Verification items for the finished model (mm, model axes). Round coordinates to 2 decimals unless told otherwise and drop trailing zeros. Order: outer loops, then holes, each group sorted by start corner. A loop starts at its lowest first (then second) coordinate and runs counter-clockwise, first axis right, second up. Notation, with made-up numbers: M -22,71 L 20,71 A30 ccw 20,108 Z; hole C 68.25,80 d3. An arc over 180 degrees is marked long. Use CSV: the item, a comma, the result in double quotes. Start each with the question number.
Q1. Sectioned sample at D-D (z = -51). Enter the section's corners in (x, y).
Q2. Mould release check, pull along X, two halves, no side actions. Record for faces 1 (the face through (-10.867, 82.767, -77.244)), 2 (the face through (0.501, 76.326, 14.743)), 3 (the face through (-25.94, 68.03, 34.57)): +X half, -X half, draft (parallel to the pull), parting line (faces both ways), or undercut.
Q3. Sectioned sample at C-C (y = 8.5). Enter the section's corners in (x, z).
Q4. Sectioned sample at A-A (x = 0). Enter the section's corners in (y, z), and give its area (3 significant figures).
Q5. Gauge pin test, flat ends, axial feed: pin 1 Ø1 at (y, z) = (43, -75) entering from +X; pin 2 Ø10 at (x, z) = (42.5, -95.5) entering from +Y; pin 3 Ø10 at (y, z) = (-30, -48) entering from -X. Record the tip position at first contact, or that the pin passes through.
Q6. Sectioned sample at B-B (y = -23). Enter the section's corners in (x, z).
Q7. Scan lines: line 1 (Y direction, x = -9.5, z = -155); line 2 (Y direction, x = 0, z = -107.5); line 3 (Y direction, x = -24, z = -144). Record each from-to range of solid material in increasing order.
```python
from build123d import *

# Parameters (mm, degrees)
SKETCH1_R                = 83.4771
SKETCH1_R_2              = 72.5043
BOSS_EXTRUDE1_DEPTH      = 203.2
BOSS_EXTRUDE1_DEPTH_BACK = 177.8
SKETCH8_W                = 2032
SKETCH8_H                = 2032
CUT_EXTRUDE10_DEPTH      = 304.8
SKETCH17_W               = 203.2
SKETCH17_H               = 508
CUT_EXTRUDE14_DEPTH      = 152.4
SKETCH18_R               = 25.4
CUT_EXTRUDE15_DEPTH      = 238.393289234


with BuildPart() as part:
    # Sketch1 → Boss-Extrude1 (new body, two sides)
    with BuildSketch(Plane.XY) as boss_extrude1_sk:
        Circle(SKETCH1_R)
        Circle(SKETCH1_R_2, mode=Mode.SUBTRACT)
    extrude(amount=BOSS_EXTRUDE1_DEPTH)
    extrude(boss_extrude1_sk.sketch, amount=-BOSS_EXTRUDE1_DEPTH_BACK)

    # Sketch8 → Cut-Extrude10 (cut)
    with BuildSketch(Plane(origin=(0, 0, 0), x_dir=(-1, 0, 0), z_dir=(0, 0.866025404, -0.5))):
        Rectangle(SKETCH8_W, SKETCH8_H)
    extrude(amount=-CUT_EXTRUDE10_DEPTH, mode=Mode.SUBTRACT)

    # Sketch17 → Cut-Extrude14 (cut)
    with BuildSketch(Plane(origin=(0, 65.991135768, 38.1), x_dir=(-1, 0, 0), z_dir=(0, 0.866025404, 0.5))):
        Rectangle(SKETCH17_W, SKETCH17_H)
    extrude(amount=CUT_EXTRUDE14_DEPTH, mode=Mode.SUBTRACT)

    # Sketch18 → Cut-Extrude15 (cut, through all)
    with BuildSketch(Plane(origin=(0, 65.991135768, 38.1), x_dir=(1, 0, 0), z_dir=(0, 0.866025404, 0.5))):
        Circle(SKETCH18_R)
    extrude(amount=-CUT_EXTRUDE15_DEPTH, mode=Mode.SUBTRACT)


solid = part.part
```
Verdict:
1,outline,"M -78.11,-29.44 L -66.26,-29.44 A72.5 cw long 66.26,-29.44 L 78.11,-29.44 A83.48 ccw long Z"
2,face 1,"parting line"
2,face 2,"undercut"
2,face 3,"draft"
3,outline,"M -83.04,-177.8 L -72,-177.8 L -72,14.72 L -83.04,14.72 Z; M 72,-177.8 L 83.04,-177.8 L 83.04,14.72 L 72,14.72 Z"
4,outline,"M -83.48,-177.8 L -72.5,-177.8 L -72.5,-125.58 L -83.48,-144.59 Z; M 72.5,-177.8 L 83.48,-177.8 L 83.48,7.81 L 78.69,16.1 L 72.5,12.53 Z"
4,area,"2,570 mm²"
5,pin 1,"stops at x = 71.85"
5,pin 2,"stops at y = 74.58"
5,pin 3,"stops at x = -79.65"
6,outline,"M -80.25,-177.8 L -68.76,-177.8 L -68.76,-39.84 L -80.25,-39.84 Z; M 68.76,-177.8 L 80.25,-177.8 L 80.25,-39.84 L 68.76,-39.84 Z"
7,line 1,"y = -82.93 to -71.88, 71.88 to 82.93"
7,line 2,"y = 72.5 to 83.48"
7,line 3,"y = -79.95 to -68.42, 68.42 to 79.95"
